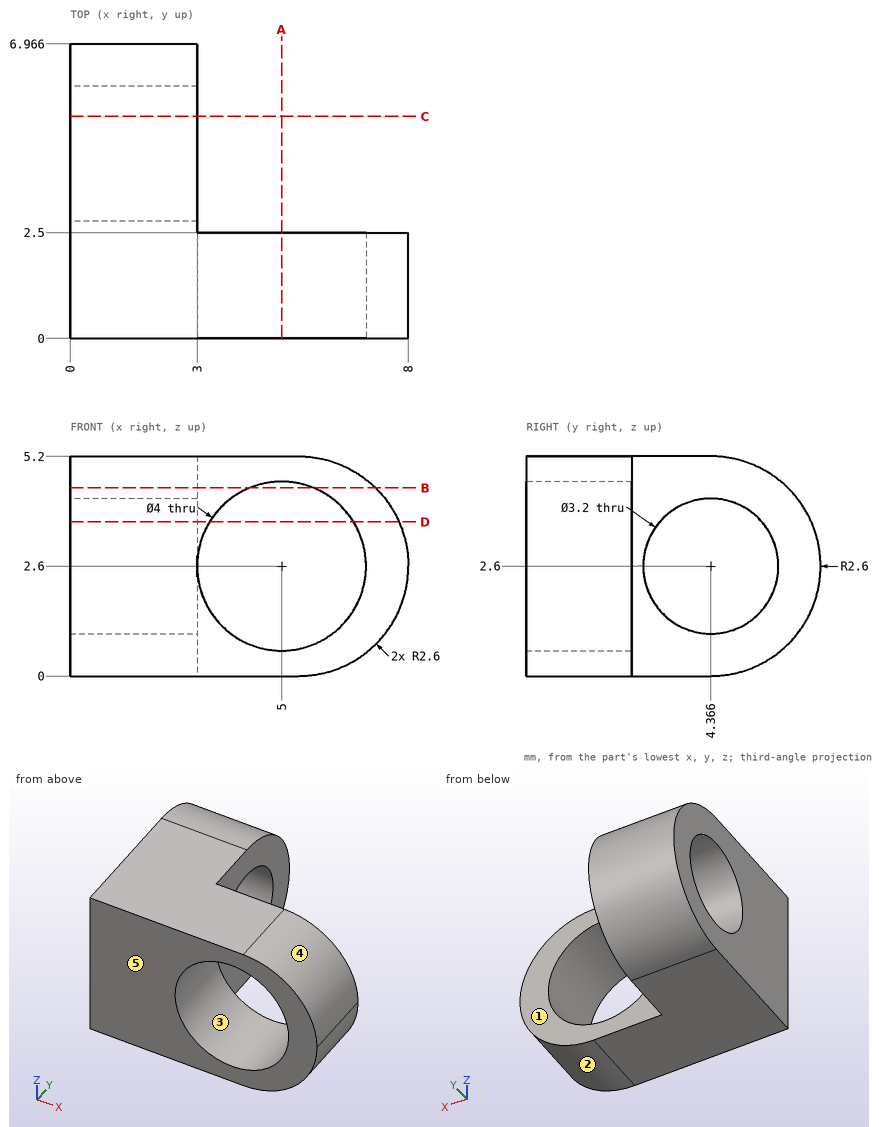
The figure shows three views and two pictorial views of one solid part (mm, origin at its lowest corner). Answer the questions. A direction names the side the tool comes from. Give positions to 0.01 mm unless a question says otherwise; leave off trailing zeros. Write each loop counter-clockwise with the first axis right and the second up, starting at its lowest first coordinate (ties: lowest second). Pieces come first, ordered by that corner, then holes. Notation, with made-up numbers: (-12, 20) -> (22, 20) arc R33 ccw to (22, 53) -> close; hole circle Ø11 at (58, -28.75). An arc over 180 degrees is marked (long way). Use one line per item in the form item = value.
1) Straight lines are drawn through the part: probe 1 along Y at (x, z) = (1.5, 2.55) (1 decimal); probe 2 along X at (y, z) = (0.8, 2.6); probe 3 along X at (y, z) = (4.25, 4.3). For each, find the intervals that lie inside material, in ascending order.
Result:
probe_1 = 0 to 2.8, 6 to 7
probe_2 = 0 to 3, 7 to 8
probe_3 = 0 to 3
2) A tool of negligible diameter and unlimited length cuts with its end or side. For the marked faces 1 and 2, from which of +Z, -Z, +X, -X, +Y, -Y can it reach the whole face along a straight path? Write none if from no direction.
Result:
face_1 = +Z, -Z, +X, +Y
face_2 = -Z, +X, +Y, -Y
3) Each of these flat-tipped pins is pushed along its axis until it touches: P1, Ø2, axis at x = 7, y = 5, coming from the -Z side; P2, Ø2, axis at y = 5.5, z = 3, coming from the +X side. Where does it stop, or does it pass through?
Result:
P1 = through
P2 = 3
4) For a pull along Z with two mould halves and no side action, classify the marked faces 3, 4 and 5 as +Z half, -Z half, draft (parallel to the pull), parting line (faces both ways), or undercut.
Result:
face_3 = undercut
face_4 = +Z half
face_5 = draft
5) Section D-D on z = 3.65 is taken. Write down the section's boundary in (x, y), plus the area to 3 significant figures.
Result:
outline = (0, 0) -> (3.3, 0) -> (3.3, 2.5) -> (3, 2.5) -> (3, 3.16) -> (0, 3.16) -> close; (0, 5.57) -> (3, 5.57) -> (3, 6.74) -> (0, 6.74) -> close; (6.7, 0) -> (7.78, 0) -> (7.78, 2.5) -> (6.7, 2.5) -> close
area = 16.4 mm²
6) Section A-A on x = 5 is taken. Write down the section's boundary in (y, z).
Result:
outline = (0, 0) -> (2.5, 0) -> (2.5, 0.6) -> (0, 0.6) -> close; (0, 4.6) -> (2.5, 4.6) -> (2.5, 5.2) -> (0, 5.2) -> close
7) Section B-B on z = 4.45 is taken. Write down the section's boundary in (x, y).
Result:
outline = (0, 0) -> (4.24, 0) -> (4.24, 2.5) -> (3, 2.5) -> (3, 6.19) -> (0, 6.19) -> close; (5.76, 0) -> (7.23, 0) -> (7.23, 2.5) -> (5.76, 2.5) -> close
8) Section C-C on y = 5.25 is taken. Write down the section's boundary in (x, z) (1 decimal).
Result:
outline = (0, 0.2) -> (3, 0.2) -> (3, 1.3) -> (0, 1.3) -> close; (0, 3.9) -> (3, 3.9) -> (3, 5) -> (0, 5) -> close
